```python
from build123d import *

# Parameters (mm, degrees)
F0_R     = 11.5
F1_DEPTH = 15
F2_ANGLE = 90
F3_R     = 10


with BuildPart() as f1:
    # F0 (on Front) → F1 (new body)
    with BuildSketch(Plane.XZ):
        Polygon((-81.4494020062, -100.8784402028), (252.5822216817, -100.8784402028), (252.5822216817, 514.1215597972), (35.2907867508, 548.5371421061), (35.2907867508, 433.5371421061), (104.0274621586, 420.2982050686), (56.4236834155, 68.4323046706), (-81.4494020062, 44.1215597972), align=None)
        with Locations((13.5479746163, -13.94874061)):
            Circle(F0_R, mode=Mode.SUBTRACT)
    extrude(amount=F1_DEPTH)


with BuildPart() as f1_1:
    # F2: moved
    add(f1.part.rotate(Axis((252.5822216817, -15, 206.6215597972), (0, 0, -1)), F2_ANGLE))

    # F3
    f3_edges = [f1_1.edges().sort_by_distance(p)[0] for p in [
        (260.082222, 202.291435, 548.537142),
        (260.082222, 202.291435, 433.537142),
        (260.082222, 133.55476, 420.298205),
        (260.082222, 181.158538, 68.432305),
        (260.082222, 319.031624, 44.12156),
        (260.082222, 319.031624, -100.87844),
    ]]
    fillet(f3_edges, radius=F3_R)


solid = f1_1.part
```
The listing builds one solid part. Answer for the finished solid, in the listing's coordinates (mm). A direction names the side the tool comes from. Coordinates: 2 decimals unless noted, no trailing zeros. Write each loop counter-clockwise with the first axis right and the second up, starting at its lowest first coordinate (ties: lowest second). Pieces come first, ordered by that corner, then holes.
Q1. Given P1, Ø1.5, axis at x = 264.5, z = 334, coming from the +Y side; P2, Ø3, axis at x = 263.5, y = 210, coming from the +Z side; P3, Ø1, axis at x = 265, z = 277.5, coming from the +Y side, each flat-ended and moving along its own axis, determine where each tip first touches the part or whether it passes through.
Returned:
P1: stops at y = 145.33
P2: stops at z = 63.61
P3: stops at y = 152.94
Q2. Section A-A, the plane x = 257 is taken. Write down the section's boundary in (y, z), then the cut area to 3 significant figures.
Returned:
outline: (-15, -100.88) - (309.03, -100.88) arc R10 ccw to (319.03, -90.88) - (319.03, 35.73) arc R10 ccw to (310.77, 45.58) - (188.35, 67.16) arc R10 cw to (180.18, 75.67) - (134.82, 410.93) arc R10 cw to (142.84, 422.09) - (194.18, 431.98) arc R10 ccw to (202.29, 441.79) - (202.29, 536.83) arc R10 ccw to (190.73, 546.71) - (-15, 514.12) - close; hole circle Ø23 at (224.03, -13.95)
area: 139,000 mm2
Q3. Section B-B, the plane z = 54.5 is taken. Write down the section's boundary in (x, y), then the cut area to 3 significant figures.
Returned:
outline: (252.58, -15) - (267.58, -15) - (267.58, 260.17) - (252.58, 260.17) - close
area: 4,130 mm2
Q4. Find the intervals of material crossed by line 1 along Z through (x, y) = (258.75, 222.5); line 2 along Y through (x, z) = (259, 182); line 3 along Y through (x, z) = (266, 298), in increasing order.
Returned:
line 1: z = -100.88 to -25.35, -2.55 to 61.14
line 2: y = -15 to 165.79
line 3: y = -15 to 150.1
Q5. Section C-C, the plane y = 251 is taken. Write down the section's boundary in (x, z).
Returned:
outline: (252.58, -100.88) - (267.58, -100.88) - (267.58, 56.12) - (252.58, 56.12) - close
Q6. Which of the six approach directions +Z, -Z, +X, -X, +Y, -Y give full straight-line access (tool end or side, diameter ignored) to faces 1 (the flat face through (267.582, 117, 228)), 2 (the flat face through (260.19, 168.87, 427.1))?
Returned:
face 1: +Z, -Z, +X, +Y, -Y
face 2: +X, -X, +Y
Q7. The mould has two halves that part along Z. Classify faces 3 (the flat face through (260, 202.291, 490)), 4 (the cylindrical face through (260.187, 213.065, -10.494)), 5 (the flat face through (260.187, 157.183, 245.646)), 6 (the flat face through (260, 149, -100.878)): released by +Z, released by -Z, zero draft, split by the parting line, or undercut.
Returned:
face 3: zero draft
face 4: undercut
face 5: undercut
face 6: released by -Z
